For this review, take the finished solid that the model builds, in its own axes (mm). Give positions to 0.01 mm unless a question says otherwise; leave off trailing zeros.
Item 1: For probe 1 along Y at (x, z) = (0, 173); probe 2 along Z at (x, y) = (117.5, 30); probe 3 along X at (y, z) = (0, 168), list the stretches that pass through material, from the lowest coordinate up.
Item 2: Consider section A-A (x = 9). Give the number of separate pieces and of enclosed holes in the cut face, plus the area to 3 significant figures.
Item 3: For P1, Ø12, axis at x = 48.5, y = -4, coming from the -Z side; P2, Ø11, axis at y = 1.5, z = 89, coming from the -X side, all flat-tipped, find the tip position at first contact; note any pin that passes through.
Autodesk Fusion 360 part; units mm, degrees
sketch "スケッチ1" plane through (0, 0, 0) normal (0, 0, 1) x (1, 0, 0)
  circle A0 centre (0, 0) radius 76
  line L0 (-25, 0) -> (125, 0)
  circle A1 centre (120, 0) radius 5
  ellipse E0 centre (0, 0) end of major axis (125, 0) minor radius 90
  line L1 (-125, 0) -> (125, 0)
  line L2 (0, -90) -> (0, 90)
  ellipse E1 centre (0, 0) end of major axis (115, 0) minor radius 80
  line L3 (-115, 0) -> (115, 0)
  line L4 (0, -80) -> (0, 80)
  circle A2 centre (0, 85) radius 5
  circle A3 centre (0, -85) radius 5
  line L5 (120, 0) -> (115, 0)
  line L6 (120, 5) -> (120, 0)
  line L7 (115, 5) -> (125, 5)
  line L8 (125, 5) -> (125, -5)
  line L9 (125, -5) -> (115, -5)
  line L10 (115, -5) -> (115, 5)
  dimension "d1" = 152
  dimension "d2" = 150
extrude "押し出し1" add sketch "スケッチ1" along normal blind 141 contours A0 L0 L1 L2 L3 L4 | A0 L0 L1 L2 L3 L4 | A0 L0 L1 L2 L3 L4 | A0 L0 L1 L2 L3 L4 makes body 1
extrude "押し出し2" add sketch "スケッチ1" along normal blind 3 separate body contours E0 E1 A3 L9 L10 | E0 E1 A2 L7 L10 | L2 A2 | L2 A2 | L2 A3 | L2 A3 makes body 2 at (30.5782, -83.5354, 0)
sketch "スケッチ2" plane through (0, 0, 0) normal (0, 1, 0) x (1, 0, 0)
  line L0 (0, -170) -> (100, -170)
  line L1 (120, -150) -> (120, 0)
  arc A0 (100, -170) -> (120, -150) centre (100, -150) ccw
  line L2 (0, -170) -> (0, -175)
  line L3 (0, -175) -> (100, -175)
  line L4 (100, -175) -> (100, -165)
  line L5 (100, -165) -> (0, -165)
  line L6 (0, -165) -> (0, -175)
  circle A1 centre (100, -150) radius 15
  circle A2 centre (100, -150) radius 25
  line L7 (125, -150) -> (115, -150)
  line L8 (115, -150) -> (115, 0)
  line L9 (115, 0) -> (125, 0)
  line L10 (125, 0) -> (125, -150)
  dimension "d11" = 20
  dimension "d24" = 5
  dimension "d25" = 100
  dimension "d26" = 10
ref_plane "作業平面1" through (0, 0, 170) normal (0, 0, 1) x (1, 0, 0)
sketch "スケッチ3" plane through (0, 0, 170) normal (0, 0, 1) x (1, 0, 0)
  circle A0 centre (0, 0) radius 3
  circle A1 centre (0, 0) radius 5
  circle A2 centre (0, 0) radius 2.5
  line L0 (0, 0) -> (-5, 0)
  line L1 (0, 0) -> (-2.5, 4.3301)
  line L2 (0, 0) -> (-2.5, -4.3301)
  circle A3 centre (-1.875, 3.2476) radius 1.25
  circle A4 centre (-1.875, -3.2476) radius 1.25
  line L3 (0, 0) -> (5, 0)
  line L4 (0, 0) -> (0, 5)
  line L5 (0, 0) -> (0, -5)
  arc A5 (0, 3) -> (-1.25, 2.1651) centre (-0.2231, 1.9809) ccw
  arc A6 (-1.25, -2.1651) -> (0, -3) centre (-0.2231, -1.9809) ccw
  dimension "d17" = 6
  dimension "d18" = 10
  dimension "d23" = 5
extrude "押し出し4" add sketch "スケッチ3" along normal mid plane 10 separate body contours A0 A1 L3 L5 | A0 A1 L3 L4 | A1 A3 L4 A5 | A0 A5 | A0 A6 | A1 A4 L5 A6 | A0 L1 A5 | A0 L1 A3 | A0 L2 A4 | A0 L2 A6 | A0 L1 A3 | A0 L1 A3 | A0 L2 A4 | A0 L2 A4 makes body 3
extrude "押し出し6" add sketch "スケッチ2" along normal mid plane 10 contours L0 L5 L6 A2 | L0 L2 L3 L6 A2 | L0 L4 L5 A2 | L0 L4 A2 | A0 L4 A1 L7 | A0 L4 A2 L7 | L1 A2 L7 L8 | L1 A2 L7 | L1 A2 L8 L9 | L1 A2 L9 L10 bodies 3 2
extrude "押し出し5" cut sketch "スケッチ3" along normal mid plane 10 contours A0 A2 L3 L4 | A0 A2 L3 L5 | A0 A2 A3 L4 | A0 A6 | A0 A2 A4 L5 | A2 L3 L4 | A2 L3 L5 | A3 A5 | A2 L1 L4 | A4 A6 bodies 3
extrude "押し出し7" cut sketch "スケッチ1" along normal blind 175 contours E0 L8 L9 | E0 L7 L8 bodies 3
sketch "スケッチ4" plane through (0, 0, 0) normal (0, 0, 1) x (1, 0, 0)
  circle A0 centre (85, 0) radius 3
  circle A1 centre (75, 0) radius 3
  dimension "d66" = 6
  dimension "d68" = 6
extrude "押し出し8" add sketch "スケッチ4" along normal blind 150 separate body makes body 4 at (85.8125, 2.8879, 100) makes body 5 at (75.8125, 2.8879, 100)
sketch "スケッチ5" plane through (0, 0, 150) normal (0, 0, 1) x (-1, 0, 0)
  circle A0 centre (-85, 0) radius 3
  circle A1 centre (-75, 0) radius 3
  circle A2 centre (-85, 0) radius 1.5
  circle A3 centre (-75, 0) radius 1.6
  dimension "d69" = 3
  dimension "d70" = 3.2
extrude "押し出し9" add sketch "スケッチ5" along normal blind 3 contours A2 bodies 4
extrude "押し出し10" cut sketch "スケッチ5" against normal blind 3 contours A3 bodies 5
sketch "スケッチ6" plane through (0, 0, 0) normal (0, 0, 1) x (1, 0, 0)
  circle A0 centre (0, 0) radius 60
  circle A1 centre (0, 0) radius 55
  circle A2 centre (0, 0) radius 25
  line L0 (0, 0) -> (0, 60)
  line L1 (2.5, 55) -> (2.5, 0)
  line L2 (2.5, 0) -> (-2.5, 0)
  line L3 (-2.5, 0) -> (-2.5, 55)
  line L4 (1.25, -2.1651) -> (-46.3814, -29.6651)
  line L5 (-48.8814, -25.3349) -> (-1.25, 2.1651)
  line L6 (-1.25, 2.1651) -> (1.25, -2.1651)
  line L7 (1.25, 2.1651) -> (48.8814, -25.3349)
  line L8 (46.3814, -29.6651) -> (-1.25, -2.1651)
  line L9 (-1.25, -2.1651) -> (1.25, 2.1651)
  circle A3 centre (0, 0) radius 3
  dimension "d41" = 50
  dimension "d43" = 5
  dimension "d45" = 360
  dimension "d48" = 6
extrude "押し出し11" add sketch "スケッチ6" along normal blind 3 separate body contours A1 A2 L0 L1 | A1 A2 L0 L3 | A0 | A2 L0 L3 A3 | A2 L0 L1 A3 | A1 A2 L4 L5 | L0 L1 L7 L9 A3 | L0 L3 L5 L6 A3 | A1 A2 L7 L8 | A2 L4 L5 A3 | L1 L2 L7 L9 | L2 L3 L4 L5 L8 L9 A3 | L2 L3 L5 L6 | L1 L2 L4 L6 L7 L8 A3 | L4 L6 L8 L9 | A2 L7 L8 A3 makes body 6
extrude "押し出し12" add sketch "スケッチ6" along normal blind 13 contours L0 L1 L7 L9 A3 | L0 L3 L5 L6 A3 | L1 L7 A3 | L3 L5 A3 | L1 L2 L7 L9 | L2 L3 L4 L5 L8 L9 A3 | L2 L3 L5 L6 | L1 L2 L4 L6 L7 L8 A3 | L4 L6 L8 L9 | L4 L8 A3 bodies 6
ref_plane "作業平面2" through (0, 0, 23) normal (0, 0, 1) x (1, 0, 0)
sketch "スケッチ7" plane through (0, 0.0029, 23) normal (0, 0, 1) x (1, 0, 0)
  circle A0 centre (0, 0) radius 25
  line L0 (0, 0) -> (25, 0) construction
  line L1 (0, 0) -> (26.2494, 0) construction
  line L2 (0, 0) -> (28.4476, 0) construction
  circle A1 centre (-20.7846, -12) radius 1
  circle A2 centre (20.7846, -12) radius 1
  circle A3 centre (0, 24) radius 1
  dimension "d61" = 2
  dimension "d62" = 2
  dimension "d63" = 2
sketch "スケッチ8" plane through (0, 0, 13) normal (0, 0, 1) x (-1, 0, 0)
  circle A0 centre (0, 0) radius 3
  circle A1 centre (0, 0) radius 3
loft "ロフト1" add profiles "スケッチ8", "スケッチ7" section 1 section 2 contours A3 bodies 6
loft "ロフト2" add profiles "スケッチ8", "スケッチ7" section 1 section 2 contours A1 bodies 6
loft "ロフト3" add profiles "スケッチ8", "スケッチ7" section 1 section 2 contours A2 bodies 6
extrude "押し出し13" add sketch "スケッチ7" against normal blind 20 contours A3 | A1 | A2 bodies 6
hidden bodies 1 4 5 6
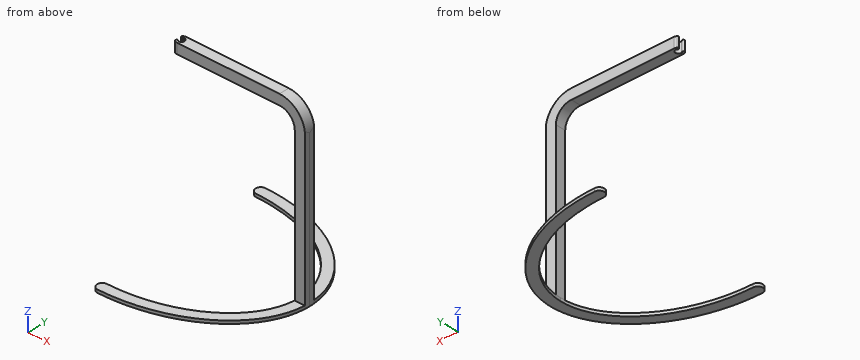
Resolved:
1. probe 1: y = -5 to -3, 3 to 5
1. probe 2: z = 0 to 3
1. probe 3: x = 3 to 117.35
2. separate pieces: 3
2. enclosed holes: 0
2. area: 160 mm2
3. P1: stops at z = 165
3. P2: stops at x = 115
